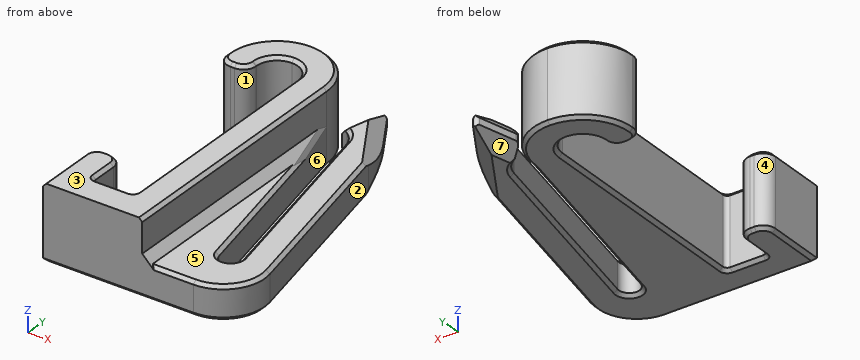
Autodesk Fusion 360 part; units mm, degrees
sketch "Sketch2" plane through (0, 0, 0) normal (0, 0, 1) x (1, 0, 0)
  line L0 (0, 0) -> (5, 0)
  line L1 (5, 0) -> (5, -30.1)
  line L2 (5, -30.1) -> (0, -30.1)
  line L3 (0, -30.1) -> (0, 0)
  line L4 (-3.5, -33.6) -> (8.5, -33.6)
  line L5 (8.5, -33.6) -> (8.5, 3.5)
  line L6 (8.5, 3.5) -> (-3.5, 3.5)
  line L7 (-3.5, 3.5) -> (-3.5, -33.6)
  line L8 (-3.5, -25.1) -> (0, -25.1)
  line L9 (-3.5, -4.1) -> (0, -4.1)
  dimension "d12" = 30.1
  dimension "d13" = 5
  dimension "d22" = 3.5
  dimension "d23" = 3.5
  dimension "d24" = 3.5
  dimension "d25" = 3.5
  dimension "d26" = 21
  dimension "d27" = 5
extrude "Extrude1" add sketch "Sketch2" along normal blind 9 contours L0 L1 L2 L3 L4 L5 L6 L7 L8 L9
fillet "Fillet1" radius 2.5 2 edges at (5, 0, 4.5) (0, 0, 4.5)
fillet "Fillet1" radius 6 2 edges at (8.5, 3.5, 4.5) (-3.5, 3.5, 4.5)
fillet "Fillet1" radius 1.5 4 edges at (0, -4.1, 4.5) (-3.5, -4.1, 4.5) (0, -25.1, 4.5) (-3.5, -25.1, 4.5)
fillet "Fillet1" radius 0.5 2 edges at (0, -30.1, 4.5) (5, -30.1, 4.5)
sketch "Sketch3" plane through (0, 0, 0) normal (0, 0, -1) x (1, 0, 0)
  arc A0 (-3.5, 26.6) -> (-2, 25.1) centre (-2, 26.6) ccw
  line L0 (-2, 25.1) -> (-1.5, 25.1)
  arc A1 (-1.5, 25.1) -> (0, 26.6) centre (-1.5, 26.6) ccw
  line L1 (0, 26.6) -> (0, 29.6)
  line L2 (0.5, 30.1) -> (4.5, 30.1)
  line L3 (5, 29.6) -> (5, 2.5)
  arc A2 (0, 2.5) -> (5, 2.5) centre (2.5, 2.5) ccw
  line L4 (0, 2.5) -> (0, 2.6)
  arc A3 (0, 2.6) -> (-1.5, 4.1) centre (-1.5, 2.6) ccw
  line L5 (-1.5, 4.1) -> (-2, 4.1)
  arc A4 (-2, 4.1) -> (-3.5, 2.6) centre (-2, 2.6) ccw
  line L6 (-3.5, 2.6) -> (-3.5, 2.5)
  arc A5 (-3.5, 2.5) -> (8.5, 2.5) centre (2.5, 2.5) ccw
  line L7 (8.5, 2.5) -> (8.5, 33.6)
  line L8 (8.5, 33.6) -> (-3.5, 33.6)
  line L9 (-3.5, 33.6) -> (-3.5, 26.6)
  line L10 (8.5, 27.6) -> (16.0491, 27.6) construction
  line L11 (13.5, 27.6) -> (8.5, 2.5)
  line L12 (16.0491, 27.6) -> (10.5511, 0)
  line L13 (0, 0) -> (10.5511, 0) construction
  line L14 (19.6179, 27.6) -> (14.4496, 1.6553)
  line L15 (8.402, 0) -> (9.8492, -5.9212)
  line L16 (8.402, 0) -> (10.8809, 1.6553)
  line L17 (14.4496, 1.6553) -> (9.8492, -5.9212)
  line L18 (14.4496, 1.6553) -> (10.8809, 1.6553) construction
  arc A6 (19.6179, 27.6) -> (14.6952, 33.6) centre (14.6952, 28.5806) ccw
  line L19 (14.6952, 33.6) -> (8.5, 33.6)
  line L20 (8.5, 2.5) -> (8.002, 0)
  line L21 (19.6179, 27.6) -> (16.0491, 27.6) construction
  circle A7 centre (14.7259, 27.3558) radius 1.25
  arc A8 (0.5, 30.1) -> (0, 29.6) centre (0.5, 29.6) ccw
  arc A9 (5, 29.6) -> (4.5, 30.1) centre (4.5, 29.6) ccw
  dimension "d36" = 2.5
  dimension "d37" = 2.5
  dimension "d38" = 5
  dimension "d39" = 3.5
  dimension "d40" = 45
  dimension "d41" = 110
  dimension "d44" = 20
  dimension "d45" = 0.4
extrude "Extrude2" add sketch "Sketch3" against normal blind 4 contours L7 L11 L12 L14 L15 L16 L17 A6 L19 A7
chamfer "Chamfer1" distance 1 angle 45 1 edges at (8.5, -18.05, 4)
chamfer "Chamfer4" distance 1.6 angle 45 4 edges at (9.1256, 2.9606, 4) (12.1494, 2.133, 4) (12.1494, 2.133, 0) (9.1256, 2.9606, 0)
fillet "Fillet3" radius 0.4 1 edges at (9.8492, 5.9212, 2)
fillet "Fillet3" radius 17 1 edges at (14.4496, -1.6553, 2)
fillet "Fillet3" radius 3 1 edges at (10.8809, -1.6553, 2)
fillet "Fillet3" radius 0.65 1 edges at (8.402, 0, 2)
chamfer "Chamfer5" distance 0.4 angle 45 9 edges at (18.5757, -31.7643, 4) (17.4907, -16.9216, 4) (12.0976, -33.6, 4) (11.5, -17.56, 4) (9.8327, -0.9554, 4) (10.6754, -1.7927, 4) (13.5377, -14.9928, 4) (14.9701, -28.5817, 4) (9, -5.01, 4.5)
chamfer "Chamfer5" distance 0.4 angle 45 24 edges at (17.4907, -16.9216, 0) (5.5976, -33.6, 0) (18.5757, -31.7643, 0) (-3.5, -30.1, 0) (2.5, 3.5, 0) (-3.5, -2.55, 0) (-3.0607, -3.6607, 0) (-1.75, -4.1, 0) (-0.4393, -3.6607, 0) (0, -2.55, 0) (2.5, 0, 0) (5, -16.05, 0) (4.8536, -29.9536, 0) (2.5, -30.1, 0) (0.1464, -29.9536, 0) (0, -28.1, 0) (-0.4393, -25.5393, 0) (-1.75, -25.1, 0) (-3.0607, -25.5393, 0) (11, -15.05, 0) (9.8327, -0.9554, 0) (10.6754, -1.7927, 0) (13.5377, -14.9928, 0) (14.9701, -28.5817, 0)
chamfer "Chamfer5" distance 0.4 angle 45 17 edges at (2.5, 0, 9) (0, -2.55, 9) (-0.4393, -3.6607, 9) (-1.75, -4.1, 9) (-3.0607, -3.6607, 9) (-3.5, -2.55, 9) (2.5, 3.5, 9) (8.5, -18.05, 9) (-3.5, -30.1, 9) (-3.0607, -25.5393, 9) (-1.75, -25.1, 9) (-0.4393, -25.5393, 9) (0, -28.1, 9) (0.1464, -29.9536, 9) (2.5, -30.1, 9) (4.8536, -29.9536, 9) (5, -16.05, 9)
equation "slot_height = 30.1 mm"
equation "slot_width = 5 mm"
equation "hook_offset = 2.5 mm"
equation "hook_slot = 2.5 mm"
equation "track_gap = 21 mm"
equation "body_width = 3.5 mm"
equation "d22 = body_width"
equation "d23 = body_width"
equation "d24 = body_width"
equation "d25 = body_width"
equation "d26 = track_gap"
equation "d36 = hook_offset"
equation "d37 = hook_slot"
equation "d39 = body_width"
equation "d40 = Angular Dimension-2"
equation "d41 = Angular Dimension-3"
equation "d44 = Angular Dimension-4"
Input: part model. Units: mm. Frame: model coordinates. Face numbers are marked on the shaded views. A direction names the side the tool comes from. Give positions to 0.01 mm unless a question says otherwise; leave off trailing zeros. Loops run counter-clockwise (first coordinate to the right, second up) from the corner with the lowest first, then second, coordinate; pieces in that order, holes last. Notation, with made-up numbers: (9, -25.75) -> (25, -25.75) arc R13 cw to (25, -20.75) -> close; hole circle Ø7 at (83, 21). An arc over 180 degrees is marked (long way). Use a Markdown table: item, result.
Q1. Pull-direction query (X, two-part tool) for the marked faces 1, 2 and 3; classes: pulls with the +X half, pulls with the -X half, needs draft (parallel to the pull), parting line crosses it, or undercut.
Entries:
| item | result |
|---|---|
| face 1 | undercut |
| face 2 | pulls with the +X half |
| face 3 | needs draft |
Q2. First-contact query: P1, Ø2, axis at x = 3, z = 3.5, coming from the +Y side; P2, Ø1, axis at y = -4.5, z = 6.5, coming from the +X side; P3, Ø8, axis at x = 14.5, y = -19.5, coming from the +Z side. Flat tips, straight axial feed; report the tip coordinate or a pass-through.
Entries:
| item | result |
|---|---|
| P1 | stops at y = 3.5 |
| P2 | stops at x = 8.5 |
| P3 | stops at z = 4 |
Q3. Ray query, probe 1 along X at (y, z) = (-26.5, 8); probe 2 along X at (y, z) = (-2, 0.75); probe 3 along X at (y, z) = (-25, 7.5). Return the intervals inside material, ascending. Write a range as from..to.
Entries:
| item | result |
|---|---|
| probe 1 | x = -3.5..0, 5..8.5 |
| probe 2 | x = -3.48..0.05, 4.95..8.48, 10.8..13.66 |
| probe 3 | x = 5..8.5 |
Q4. Access query for the marked faces 4, 5, 6 and 7. Directions: +Z, -Z, +X, -X, +Y, -Y. A direction counts if a zero-diameter tool reaches every point of the face in a straight line with its end or side. Return the directions, or none.
Entries:
| item | result |
|---|---|
| face 4 | +Z, -Z, -X |
| face 5 | +Z, +X, +Y, -Y |
| face 6 | +Z, -Z |
| face 7 | -Z, +Y |
Q5. Section query A-A, the plane y = -10. Return the cut outline in (x, z), plus the area to 3 significant figures.
Entries:
| item | result |
|---|---|
| outline | (5, 0.4) -> (5.4, 0) -> (9.59, 0) -> (9.99, 0.4) -> (9.99, 3.6) -> (9.59, 4) -> (9.5, 4) -> (8.5, 5) -> (8.5, 8.6) -> (8.1, 9) -> (5.4, 9) -> (5, 8.6) -> close; (12.54, 0.4) -> (12.95, 0) -> (15.7, 0) -> (16.11, 0.4) -> (16.11, 3.6) -> (15.7, 4) -> (12.95, 4) -> (12.54, 3.6) -> close |
| area | 51.5 mm² |
